CAD build for the part. Positions are in the model's coordinates, mm. A direction names the side the tool comes from. Give positions to 0.01 mm unless a question says otherwise; leave off trailing zeros. Write each loop counter-clockwise with the first axis right and the second up, starting at its lowest first coordinate (ties: lowest second). Pieces come first, ordered by that corner, then holes. Notation, with made-up numbers: (53.5, 85.5) - (86.5, 85.5) arc R19 ccw to (86.5, 115.5) - close; hole circle Ø9 at (-29, -5). An arc over 180 degrees is marked (long way). Answer as a JSON object with one key per item and string values.
from build123d import *

# Parameters (mm, degrees)
F1_DEPTH = 1.5
F3_DEPTH = 25
F2_W     = 3
F2_H     = 2
F2_W_2   = 21
F2_H_2   = 3
F4_DEPTH = 3.5
F6_DEPTH = 127


with BuildPart() as f1:
    # F0 (on Top) → F1 (new body)
    with BuildSketch(Plane.XY):
        Polygon((0, 5.5), (0, 0), (21, 0), (21, 5.5), (18, 5.5), (18, 3), (3, 3), (3, 5.5), align=None)
    extrude(amount=F1_DEPTH)

    # F2 (on face) → F3 (join)
    with BuildSketch(Plane.XY.offset(1.5)):
        Polygon((3, 3), (0, 3), (0, 0), (21, 0), (21, 3), (18, 3), align=None)
    extrude(amount=F3_DEPTH)

    # F2 (on face) → F4 (join)
    with BuildSketch(Plane.XY.offset(1.5)):
        with Locations((1.5, 4.5)):
            Rectangle(F2_W, F2_H)
        with Locations((19.5, 4.5)):
            Rectangle(F2_W, F2_H)
        with Locations((10.5, 1.5)):
            Rectangle(F2_W_2, F2_H_2)
    extrude(amount=F4_DEPTH)

    # F5 (on face) → F6 (cut)
    with BuildSketch(Plane(origin=(0, 0, 0), x_dir=(0, -1, 0), z_dir=(-1, 0, 0))):
        Polygon((-3.5, 5), (-5.5, 5), (-3.5, 1.5), align=None)
    extrude(amount=-F6_DEPTH, mode=Mode.SUBTRACT)


solid = f1.part
(1) Flat gauge pins, fed straight in: P1, Ø1, axis at x = 17, z = 20.5, coming from the +Y side; P2, Ø0.6, axis at x = 19, y = 3.5, coming from the +Z side (3 decimals). Where does each tip first touch, or does it go through?
Answer key:
{"P1": "stops at y = 3", "P2": "stops at z = 2.025"}
(2) Pull direction Y, two halves, no side cores. Call faces 1 (the face through (10, 2, 0)), 2 (the face through (20, 5.5, 2)), 3 (the face through (1.48, 4.51, 3.27)): pulls with the +Y half, pulls with the -Y half, needs draft (parallel to the pull), parting line crosses it, or undercut.
Answer key:
{"face 1": "needs draft", "face 2": "pulls with the +Y half", "face 3": "undercut"}
(3) Saw through at D-D, the plane x = 11.5. Give the cut face in (y, z), and give its area (3 significant figures).
Answer key:
{"outline": "(0, 0) - (3, 0) - (3, 26.5) - (0, 26.5) - close", "area": "79.5 mm²"}
(4) Saw through at B-B, the plane x = 19. Give the cut face in (y, z), and give its area (4 significant figures).
Answer key:
{"outline": "(0, 0) - (5.5, 0) - (5.5, 5) - (3.5, 1.5) - (3, 1.5) - (3, 26.5) - (0, 26.5) - close", "area": "86.75 mm²"}
(5) Probe L1, parallel to Y at x = 3.5, z = 4.25; L2, parallel to Y at x = 2, z = 4.5. List the from-to ranges inside material, lowest first. Write a range as [from, to].
Answer key:
{"L1": "y = [0, 3]", "L2": "y = [0, 3], [5.21, 5.5]"}
(6) Saw through at A-A, the plane y = 4.55. Give the cut face in (x, z), and give its area (3 significant figures).
Answer key:
{"outline": "(0, 0) - (3, 0) - (3, 3.34) - (0, 3.34) - close; (18, 0) - (21, 0) - (21, 3.34) - (18, 3.34) - close", "area": "20.0 mm²"}
(7) Saw through at C-C, the plane z = 9.75. Give the cut face in (x, y), and give its area (3 significant figures).
Answer key:
{"outline": "(0, 0) - (21, 0) - (21, 3) - (0, 3) - close", "area": "63.0 mm²"}
(8) 3-axis set-ups, long thin cutter, end or side, ignore diameter. For faces 4 (the face through (0, 1, 13)), 5 (the face through (19.48, 4.51, 3.27)), 6 (the face through (3, 5, 2)): which of +Z, -Z, +X, -X, +Y, -Y reach the whole face in a straight line?
Answer key:
{"face 4": "+Z, -Z, -X, +Y, -Y", "face 5": "+Z, +X, -X", "face 6": "+Z, -Z, +Y"}
